Autodesk Inventor part; units mm, degrees
ref_plane "IDS_WORKPLANE{1}" through (-6.35, 0, 0) normal (1, 0, 0) x (0, 0, -1)
ref_plane "Work Plane2" through (-3.175, 0, 0) normal (0, 0, -1) x (1, 0, 0)
ref_plane "YZ Plane" through (0, 0, 0) normal (1, 0, 0) x (0, 1, 0)
sketch "Sketch1" plane through (0, 0, 0) normal (0, 0, 1) x (1, 0, 0)
  line L0 (-6.35, 0) -> (31.75, 0)
  line L1 (31.75, 0) -> (31.75, 3.175)
  line L2 (31.75, 3.175) -> (0, 3.175)
  line L3 (0, 3.175) -> (0, 4.7625)
  line L4 (-16.0335, 0) -> (39.7139, 0)
  line L5 (0, -0.9525) -> (0, 5.715)
  line L6 (0, 4.7625) -> (-6.35, 4.7625)
  line L7 (-6.35, 0) -> (-6.35, 4.7625)
  arc A0 (-2.5645, 0) -> (-3.302, 2.7526) centre (-8.0696, 0) ccw
  line L8 (-6.35, 2.7526) -> (-3.302, 2.7526)
  line L9 (12.7, 3.175) -> (0, 3.175) construction
  dimension "d0" = 31.75
  dimension "d1" = 6.35
  dimension "d2" = 6.35
  dimension "d5" = 9.525
  dimension "d13" = 5.5051
  dimension "d14" = 5.5051
  dimension "d15" = 3.048
revolve "Body" add sketch "Sketch1" angle 360 about axis through (-6.35, 0, 0) along (1, 0, 0) contours A0 L8 L7 L6 L3 L5 L0 | L5 L2 L1 L0
ref_plane "IDS_WORKPLANE{1}" through (-6.35, 0, 0) normal (1, 0, 0) x (0, 0, -1)
sketch "Sketch2" plane through (-6.35, 0, 0) normal (1, 0, 0) x (0, 0, -1)
  line L0 (0, -6.6675) -> (0, 6.6675)
  line L1 (6.6675, 0) -> (-6.6675, 0)
  circle A0 centre (0, 0) radius 4.7625
  line L2 (2.6768, 0.6414) -> (2.2959, 0.6414)
  line L3 (0, 0) -> (2.6768, 0.6414) construction
  line L4 (0, 0) -> (4.0727, 3.8613) construction
  line L5 (0, 0) -> (0.783, 2.6389) construction
  line L6 (0, 0) -> (1.3763, 2.3838) construction
  line L7 (0.783, 2.6389) -> (0.5925, 2.309)
  line L8 (1.8938, 1.9975) -> (1.7034, 1.6676)
  line L9 (0, 0) -> (1.8938, 1.9975) construction
  arc A1 (2.3838, 0) -> (2.2959, 0.6414) centre (0, 0) ccw
  arc A2 (1.7034, 1.6676) -> (0.5925, 2.309) centre (0, 0) ccw
  arc A3 (2.7526, 0) -> (2.6768, 0.6414) centre (0, 0) ccw
  arc A4 (1.8938, 1.9975) -> (0.783, 2.6389) centre (0, 0) ccw
  arc A5 (2.6768, 0.6414) -> (1.6232, 2.223) centre (0, 0) ccw construction
  arc A6 (2.2959, 0.6414) -> (1.7034, 1.6676) centre (0, 0) ccw construction
  line L10 (2.6768, -0.6414) -> (2.2959, -0.6414)
  line L11 (0.783, -2.6389) -> (0.5925, -2.309)
  line L12 (1.8938, -1.9975) -> (1.7034, -1.6676)
  arc A7 (2.2959, -0.6414) -> (2.3838, 0) centre (0, 0) ccw
  arc A8 (0.5925, -2.309) -> (1.7034, -1.6676) centre (0, 0) ccw
  arc A9 (2.6768, -0.6414) -> (2.7526, 0) centre (0, 0) ccw
  arc A10 (0.783, -2.6389) -> (1.8938, -1.9975) centre (0, 0) ccw
  line L13 (-2.6768, 0.6414) -> (-2.2959, 0.6414)
  line L14 (-0.783, 2.6389) -> (-0.5925, 2.309)
  line L15 (-1.8938, 1.9975) -> (-1.7034, 1.6676)
  arc A11 (-2.2959, 0.6414) -> (-2.3838, 0) centre (0, 0) ccw
  arc A12 (-0.5925, 2.309) -> (-1.7034, 1.6676) centre (0, 0) ccw
  arc A13 (-2.6768, 0.6414) -> (-2.7526, 0) centre (0, 0) ccw
  arc A14 (-0.783, 2.6389) -> (-1.8938, 1.9975) centre (0, 0) ccw
  line L16 (-0.783, -2.6389) -> (-0.5925, -2.309)
  arc A15 (-1.7034, -1.6676) -> (-0.5925, -2.309) centre (0, 0) ccw
  line L17 (-1.8938, -1.9975) -> (-1.7034, -1.6676)
  arc A16 (-1.8938, -1.9975) -> (-0.783, -2.6389) centre (0, 0) ccw
  arc A17 (-2.3838, 0) -> (-2.2959, -0.6414) centre (0, 0) ccw
  line L18 (-2.6768, -0.6414) -> (-2.2959, -0.6414)
  arc A18 (-2.7526, 0) -> (-2.6768, -0.6414) centre (0, 0) ccw
  point P0 (1.3763, -2.3838)
  point P1 (-1.3763, 2.3838)
  point P2 (-1.3763, -2.3838)
  dimension "d19" = 0.6413
  dimension "d20" = 1.2827
  dimension "d21" = 33.052
  dimension "d22" = 5.5051
  dimension "d23" = 4.7676
extrude "Slot" add sketch "Sketch2" along normal up to next contours A1 L2 A3 L1 | L1 A9 L10 A7 | A17 L18 A18 L1 | L1 A13 L13 A11 | A4 L8 A2 L7 | L11 A8 L12 A10 | L14 A12 L15 A14 | A16 L17 A15 L16
fillet "Fillet1" radius 0.635 1 edges at (-6.35, -4.7625, 0)
thread "Thread"
chamfer "Chamfer1" distance 0.541 distance2 0.541 1 edges at (31.75, -3.175, 0) measured on face at (31.75, -0.3658, -0.0841)
ref_plane "Work Plane2" through (-3.175, 0, 0) normal (0, 0, -1) x (1, 0, 0)
equation "\"d19\" = 0.5 * SBR"
equation "\"d20\" = SBR"
equation "\"d22\" = 1.1547 * SW"
equation "\"d23\" = SW"
equation "\"d17\" = INTI"
equation "\"d24\" = RR"
equation "\"d6\" = GEL"
equation "\"d9\" = -0.5 * SPD + 0.5 * NND"
equation "\"d10\" = GUL"
equation "\"d0\" = NLG"
equation "\"d1\" = KOH"
equation "\"d2\" = NND"
equation "\"d5\" = KOD"
equation "\"d13\" = 1.1547 * SW"
equation "\"d14\" = 1.1547 * SW"
equation "\"d15\" = INTI"
equation "\"NND\" = 6.35"
equation "\"NLG\" = 31.75"
equation "\"GEL\" = 30.38932"
equation "\"KOD\" = 9.525"
equation "\"KOH\" = 6.35"
equation "\"SPD\" = GD1"
equation "\"GUL\" = 0.54102"
equation "\"SBR\" = 1.2827"
equation "\"INTI\" = 3.048"
equation "\"d11\" = -KOH"
equation "\"SW\" = 4.76758"
equation "\"d16\" = 1.1547 * SW"
equation "\"d18\" = SW"
equation "\"RR\" = 0.635"
equation "\"TOA\" = 30deg"
equation "\"GD1\" = 5.26796"
equation "\"THREADDIA\" = 6.35"
equation "\"BDM\" = NND"
equation "\"GD\" = NND"
equation "\"GAL\" = 1.36068"
equation "\"E0\" = 5.55498"
properties part number "ANSI B18.3 - 1/4-28 UNF - 1.25" material "Steel, Mild"
Verification items for the finished model (mm, model axes). A direction names the side the tool comes from. Coordinates: 2 decimals unless noted, no trailing zeros. Write each loop counter-clockwise with the first axis right and the second up, starting at its lowest first coordinate (ties: lowest second). Pieces come first, ordered by that corner, then holes. Notation, with made-up numbers: (-6, 53.25) - (0, 53.25) arc R33 cw to (0, 91.25) - close; hole circle Ø6 at (41.5, 29.5). An arc over 180 degrees is marked (long way). Answer as a JSON object with one key per item and string values.
(1) Cross-section at A-A on x = -2. Record the cut outline in (y, z) (1 decimal), plus the area to 3 significant figures.
Report:
{"outline": "circle Ø9.5 at (0, 0)", "area": "71.3 mm^2"}
(2) Cross-section at B-B on x = 28.5. Record the cut outline in (y, z) (3 decimals).
Report:
{"outline": "circle Ø6.35 at (0, 0)"}
(3) Tool access check on faces 1 (the cylindrical face through (15.39, -0.69, 3.1)), 2 (the flat face through (-6.35, 0, -3)), 3 (the cylindrical face through (-4.75, -2.06, -1.2)). Record the directions out of +Z, -Z, +X, -X, +Y, -Y that give a thin tool (end or side, any length) a straight path to the whole face; none if there is none.
Report:
{"face 1": "+X", "face 2": "+Z, -Z, -X, +Y, -Y", "face 3": "-X"}
(4) Mould release check, pull along Z, two halves, no side actions. Record for faces 4 (the cylindrical face through (-2.9, -3.78, 2.9)), 5 (the flat face through (31.75, 0, 0)), 6 (the cylindrical face through (-4.75, -2.07, 1.18)), 7 (the cylindrical face through (-4.75, 2.07, -1.18)): pulls with the +Z half, pulls with the -Z half, needs draft (parallel to the pull), parting line crosses it, or undercut.
Report:
{"face 4": "parting line crosses it", "face 5": "needs draft", "face 6": "undercut", "face 7": "undercut"}
(5) Gauge pin test, flat ends, axial feed: pin 1 Ø4 at (x, y) = (21.5, 2.5) entering from +Z; pin 2 Ø5 at (x, z) = (22.5, -2.5) entering from -Y (3 decimals); pin 3 Ø3 at (x, y) = (4, -1) entering from +Z (3 decimals). Record the tip position at first contact, or that the pin passes through.
Report:
{"pin 1": "z = 3.14", "pin 2": "y = -3.175", "pin 3": "z = 3.175"}
(6) Thickness scan on line 1 along Z through (x, y) = (21, 0) (3 decimals); line 2 along X through (y, z) = (0.5, -4); line 3 along Z through (x, y) = (-3.5, -3.25). Record the ranges inside material, lowest first.
Report:
{"line 1": "-3.175 to 3.175", "line 2": "-6.35 to 0", "line 3": "-3.48 to 3.48"}
